from build123d import *

# Parameters (mm, degrees)
SKETCH1_R           = 1.25
BOSS_EXTRUDE1_DEPTH = 5
FILLET1_R           = 20
FILLET2_R           = 5


with BuildPart() as part:
    # Sketch1 → Boss-Extrude1 (new body)
    with BuildSketch(Plane.XY):
        with BuildLine():
            Line((32, 5), (-32, 5))
            Line((-32, 5), (-32, 59.644660941))
            ThreePointArc((-32, 59.644660941), (-30.47759065, 67.298329588), (-26.142135624, 73.786796564))
            Line((-26.142135624, 73.786796564), (-14.142135624, 85.786796564))
            ThreePointArc((-14.142135624, 85.786796564), (0, 91.644660941), (14.142135624, 85.786796564))
            Line((14.142135624, 85.786796564), (26.142135624, 73.786796564))
            ThreePointArc((26.142135624, 73.786796564), (30.47759065, 67.298329588), (32, 59.644660941))
            Line((32, 59.644660941), (32, 5))
        make_face()
        with Locations((0, 85.644660941)):
            Circle(SKETCH1_R, mode=Mode.SUBTRACT)
        with Locations((-13.102089171, 78.341561643)):
            Circle(SKETCH1_R, mode=Mode.SUBTRACT)
        with Locations((-23.708690889, 67.734959925)):
            Circle(SKETCH1_R, mode=Mode.SUBTRACT)
        with Locations((-26, 52.910996131)):
            Circle(SKETCH1_R, mode=Mode.SUBTRACT)
        with Locations((-26, 36.198039027)):
            Circle(SKETCH1_R, mode=Mode.SUBTRACT)
        with Locations((-26, 21.198039027)):
            Circle(SKETCH1_R, mode=Mode.SUBTRACT)
        with Locations((0, 11)):
            Circle(SKETCH1_R, mode=Mode.SUBTRACT)
        with Locations((-15, 11)):
            Circle(SKETCH1_R, mode=Mode.SUBTRACT)
        with Locations(Location((13.102089171, 78.341561643, 0), (0, 0, 180))):
            Circle(SKETCH1_R, mode=Mode.SUBTRACT)
        with Locations(Location((23.708690889, 67.734959925, 0), (0, 0, 180))):
            Circle(SKETCH1_R, mode=Mode.SUBTRACT)
        with Locations(Location((26, 52.910996131, 0), (0, 0, 180))):
            Circle(SKETCH1_R, mode=Mode.SUBTRACT)
        with Locations(Location((26, 36.198039027, 0), (0, 0, 180))):
            Circle(SKETCH1_R, mode=Mode.SUBTRACT)
        with Locations(Location((26, 21.198039027, 0), (0, 0, 180))):
            Circle(SKETCH1_R, mode=Mode.SUBTRACT)
        with Locations(Location((15, 11, 0), (0, 0, 180))):
            Circle(SKETCH1_R, mode=Mode.SUBTRACT)
        with BuildLine():
            Line((-22, 59.644660941), (-22, 15))
            Line((-22, 15), (22, 15))
            Line((22, 15), (22, 59.644660941))
            ThreePointArc((22, 59.644660941), (21.238795325, 63.471495264), (19.071067812, 66.715728753))
            Line((19.071067812, 66.715728753), (7.071067812, 78.715728753))
            ThreePointArc((7.071067812, 78.715728753), (0, 81.644660941), (-7.071067812, 78.715728753))
            Line((-7.071067812, 78.715728753), (-19.071067812, 66.715728753))
            ThreePointArc((-19.071067812, 66.715728753), (-21.238795325, 63.471495264), (-22, 59.644660941))
        make_face(mode=Mode.SUBTRACT)
    extrude(amount=BOSS_EXTRUDE1_DEPTH)

    # Fillet1
    fillet1_edges = [part.edges().sort_by_distance(p)[0] for p in [
        (32, 5, 2.5),
        (-32, 5, 2.5),
    ]]
    fillet(fillet1_edges, radius=FILLET1_R)

    # Fillet2
    fillet2_edges = [part.edges().sort_by_distance(p)[0] for p in [
        (22, 15, 2.5),
        (-22, 15, 2.5),
    ]]
    fillet(fillet2_edges, radius=FILLET2_R)


solid = part.part
The listing builds one solid part. Answer for the finished solid, in the listing's coordinates (mm). A direction names the side the tool comes from. Give positions to 0.01 mm unless a question says otherwise; leave off trailing zeros. Write each loop counter-clockwise with the first axis right and the second up, starting at its lowest first coordinate (ties: lowest second). Pieces come first, ordered by that corner, then holes. Notation, with made-up numbers: (-16.75, 59) -> (-5.75, 59) arc R23 cw to (-5.75, 75) -> close; hole circle Ø11 at (77.25, 83). An arc over 180 degrees is marked (long way). Use a Markdown table: item, result.
(1) Flat-ended cylindrical pins translate along their axes: P1, Ø2.5, axis at x = -5.5, z = 2.5, coming from the +Y side; P2, Ø4, axis at x = 0, y = 11, coming from the -Z side. Find the tip coordinate at first contact, or state that the pin passes through.
Return value:
| item | result |
|---|---|
| P1 | y = 91.19 |
| P2 | z = 0 |
(2) Determine the mould class of faces 1 (the cylindrical face through (25.986, 10.703, 2.535)), 2 (the cylindrical face through (21, 17, 3)), 3 (the cylindrical face through (-0.22, 91.643, 2.465)) for opening direction X: released by +X, released by -X, zero draft, split by the parting line, or undercut.
Return value:
| item | result |
|---|---|
| face 1 | released by +X |
| face 2 | undercut |
| face 3 | split by the parting line |
(3) Section C-C, the plane z = 2.5 is taken. Give the number of separate pieces and of enclosed holes in the cut face, then the cut area to 3 significant figures.
Return value:
| item | result |
|---|---|
| separate pieces | 1 |
| enclosed holes | 15 |
| area | 2,110 mm2 |
(4) For faces 4 (the flat face through (-20.23, 79.7, 2.46)), 5 (the flat face through (0, 15, 2)), determine the directions among +Z, -Z, +X, -X, +Y, -Y from which every point of the face is accessible in a straight line to the end or side of a thin tool.
Return value:
| item | result |
|---|---|
| face 4 | +Z, -Z, -X, +Y |
| face 5 | +Z, -Z |
(5) Section B-B, the plane y = 45 is taken. Determine the outline of the cut face in (x, z), then the cut area to 3 significant figures.
Return value:
| item | result |
|---|---|
| outline | (-32, 0) -> (-22, 0) -> (-22, 5) -> (-32, 5) -> close; (22, 0) -> (32, 0) -> (32, 5) -> (22, 5) -> close |
| area | 100 mm2 |
(6) Find the intervals of material crossed by probe 1 along Y at (x, z) = (0, 3.8); probe 2 along X at (y, z) = (28.5, 1.25); probe 3 along Y at (x, z) = (26.5, 1.45), in increasing order. Write a range as from..to.
Return value:
| item | result |
|---|---|
| probe 1 | 5..9.75, 12.25..15, 81.64..84.39, 86.89..91.64 |
| probe 2 | -32..-22, 22..32 |
| probe 3 | 11.23..20.05, 22.34..35.05, 37.34..51.77, 54.06..73.42 |
(7) Section D-D, the plane y = 11 is taken. Determine the outline of the cut face in (x, z).
Return value:
| item | result |
|---|---|
| outline | (-26.28, 0) -> (-16.25, 0) -> (-16.25, 5) -> (-26.28, 5) -> close; (-13.75, 0) -> (-1.25, 0) -> (-1.25, 5) -> (-13.75, 5) -> close; (1.25, 0) -> (13.75, 0) -> (13.75, 5) -> (1.25, 5) -> close; (16.25, 0) -> (26.28, 0) -> (26.28, 5) -> (16.25, 5) -> close |
(8) Section A-A, the plane x = 0 is taken. Determine the outline of the cut face in (y, z), then the cut area to 3 significant figures.
Return value:
| item | result |
|---|---|
| outline | (5, 0) -> (9.75, 0) -> (9.75, 5) -> (5, 5) -> close; (12.25, 0) -> (15, 0) -> (15, 5) -> (12.25, 5) -> close; (81.64, 0) -> (84.39, 0) -> (84.39, 5) -> (81.64, 5) -> close; (86.89, 0) -> (91.64, 0) -> (91.64, 5) -> (86.89, 5) -> close |
| area | 75.0 mm2 |
